Check sheet for the modelled part. Datum: model origin and axes. Units: mm. A direction names the side the tool comes from. Give positions to 0.01 mm unless a question says otherwise; leave off trailing zeros. Loops run counter-clockwise (first coordinate to the right, second up) from the corner with the lowest first, then second, coordinate; pieces in that order, holes last. Notation, with made-up numbers: M 64.5,49.5 L 90.5,49.5 A22 cw 90.5,66.5 Z; hole C -24.5,-6.75 d7. An arc over 180 degrees is marked long. Put each result on its own line as item: value. Start each with the question number.
```python
from build123d import *

# Parameters (mm, degrees)
SKETCH3_R           = 0.9
SKETCH3_W           = 4.2
SKETCH3_H           = 8
SKETCH3_H_2         = 6
BOSS_EXTRUDE3_DEPTH = 2


with BuildPart() as part:
    # Sketch3 → Boss-Extrude3 (new body)
    with BuildSketch(Plane.XY):
        with BuildLine():
            Line((0, 94.006448831), (0, 86.061448831))
            ThreePointArc((0, 86.061448831), (0.585786438, 84.647235269), (2, 84.061448831))
            Line((2, 84.061448831), (4, 84.061448831))
            Line((4, 84.061448831), (4, 78.061448831))
            Line((4, 78.061448831), (2, 78.061448831))
            ThreePointArc((2, 78.061448831), (0.585786438, 77.475662393), (0, 76.061448831))
            Line((0, 76.061448831), (0, 60.606448831))
            ThreePointArc((0, 60.606448831), (0.585786438, 59.192235269), (2, 58.606448831))
            Line((2, 58.606448831), (4, 58.606448831))
            Line((4, 58.606448831), (4, 50.606448831))
            Line((4, 50.606448831), (2, 50.606448831))
            ThreePointArc((2, 50.606448831), (0.585786438, 50.020662393), (0, 48.606448831))
            Line((0, 48.606448831), (0, 26.346448831))
            ThreePointArc((0, 26.346448831), (0.585786438, 24.932235269), (2, 24.346448831))
            Line((2, 24.346448831), (4, 24.346448831))
            Line((4, 24.346448831), (4, 12.346448831))
            Line((4, 12.346448831), (6, 12.346448831))
            Line((6, 12.346448831), (6, 24.346448831))
            Line((6, 24.346448831), (10.2, 24.346448831))
            Line((10.2, 24.346448831), (10.2, 12.346448831))
            Line((10.2, 12.346448831), (12.2, 12.346448831))
            Line((12.2, 12.346448831), (12.2, 24.346448831))
            Line((12.2, 24.346448831), (14.2, 24.346448831))
            ThreePointArc((14.2, 24.346448831), (15.614213562, 24.932235269), (16.2, 26.346448831))
            Line((16.2, 26.346448831), (16.2, 48.606448831))
            ThreePointArc((16.2, 48.606448831), (15.614213562, 50.020662393), (14.2, 50.606448831))
            Line((14.2, 50.606448831), (12.2, 50.606448831))
            Line((12.2, 50.606448831), (12.2, 58.606448831))
            Line((12.2, 58.606448831), (14.2, 58.606448831))
            ThreePointArc((14.2, 58.606448831), (15.614213562, 59.192235269), (16.2, 60.606448831))
            Line((16.2, 60.606448831), (16.2, 76.061448831))
            ThreePointArc((16.2, 76.061448831), (15.614213562, 77.475662393), (14.2, 78.061448831))
            Line((14.2, 78.061448831), (12.2, 78.061448831))
            Line((12.2, 78.061448831), (12.2, 84.061448831))
            Line((12.2, 84.061448831), (14.2, 84.061448831))
            ThreePointArc((14.2, 84.061448831), (15.614213562, 84.647235269), (16.2, 86.061448831))
            Line((16.2, 86.061448831), (16.2, 94.006448831))
            Line((16.2, 94.006448831), (0, 94.006448831))
        make_face()
        with Locations((6, 33.846448831)):
            Circle(SKETCH3_R, mode=Mode.SUBTRACT)
        with Locations((10.2, 33.846448831)):
            Circle(SKETCH3_R, mode=Mode.SUBTRACT)
        with Locations((2.75, 86.061448831)):
            Circle(SKETCH3_R, mode=Mode.SUBTRACT)
        with Locations((10.2, 41.166448831)):
            Circle(SKETCH3_R, mode=Mode.SUBTRACT)
        with Locations((13.45, 48.106448831)):
            Circle(SKETCH3_R, mode=Mode.SUBTRACT)
        with Locations((2.75, 92.061448831)):
            Circle(SKETCH3_R, mode=Mode.SUBTRACT)
        with Locations((13.45, 86.061448831)):
            Circle(SKETCH3_R, mode=Mode.SUBTRACT)
        with Locations((2.75, 61.106448831)):
            Circle(SKETCH3_R, mode=Mode.SUBTRACT)
        with Locations((13.45, 61.106448831)):
            Circle(SKETCH3_R, mode=Mode.SUBTRACT)
        with Locations((2.75, 75.561448831)):
            Circle(SKETCH3_R, mode=Mode.SUBTRACT)
        with Locations((13.45, 26.846448831)):
            Circle(SKETCH3_R, mode=Mode.SUBTRACT)
        with Locations((13.45, 75.561448831)):
            Circle(SKETCH3_R, mode=Mode.SUBTRACT)
        with Locations((13.45, 92.061448831)):
            Circle(SKETCH3_R, mode=Mode.SUBTRACT)
        with Locations((2.75, 26.846448831)):
            Circle(SKETCH3_R, mode=Mode.SUBTRACT)
        with Locations((6, 41.106448831)):
            Circle(SKETCH3_R, mode=Mode.SUBTRACT)
        with Locations((2.75, 48.106448831)):
            Circle(SKETCH3_R, mode=Mode.SUBTRACT)
        with Locations((8.1, 54.606448831)):
            Rectangle(SKETCH3_W, SKETCH3_H, mode=Mode.SUBTRACT)
        with Locations((8.1, 81.061448831)):
            Rectangle(SKETCH3_W, SKETCH3_H_2, mode=Mode.SUBTRACT)
    extrude(amount=BOSS_EXTRUDE3_DEPTH)


solid = part.part
```
Q1. Mould release check, pull along X, two halves, no side actions. Record for faces 1 (the face through (12.2, 55, 1)), 2 (the face through (10.2, 18, 1)), 3 (the face through (3.23, 48.87, 0.99)), 4 (the face through (4.4, 53.7, 2)): pulls with the +X half, pulls with the -X half, needs draft (parallel to the pull), parting line crosses it, or undercut.
Q2. Access from +Z, -Z, +X, -X, +Y, -Y to the whole of each face (thin tool, end or side, straight path). Record for faces 5 (the face through (4, 81, 1)), 6 (the face through (15.63, 50.005, 0.986)), 7 (the face through (10.2, 55, 1)), 8 (the face through (16.2, 90, 1)), 9 (the face through (4, 18, 1)).
Q3. Section check A-A, the plane y = 22. Record the cut outline in (x, z).
Q4. Section check B-B, the plane x = 2.75. Give the number of separate pieces and of enclosed holes in the cut face, then the cut area to 3 significant figures.
Q5. Thickness scan on line 1 along Y through (x, z) = (8, 1.75); line 2 along X through (y, z) = (16.5, 1); line 3 along Y through (x, z) = (10, 1.4). Record the ranges inside material, lowest first. Write a range as [from, to].
Q6. Depth check by flat-ended pin: P1, Ø1, axis at x = 3, z = 1, coming from the -Y side; P2, Ø0.6, axis at y = 55, z = 1, coming from the -X side; P3, Ø1.4, axis at x = 2.75, y = 48.11, coming from the +Z side; P4, Ø3, axis at x = 13.45, y = 86.06, coming from the -Z side. Enter the tip coordinate at first touch or a pass-through.
Found:
1. face 1: pulls with the +X half
1. face 2: undercut
1. face 3: undercut
1. face 4: needs draft
2. face 5: +Z, -Z, -X
2. face 6: +Z, -Z, +X
2. face 7: +Z, -Z
2. face 8: +Z, -Z, +X, +Y, -Y
2. face 9: +Z, -Z, -X, -Y
3. outline: M 4,0 L 6,0 L 6,2 L 4,2 Z; M 10.2,0 L 12.2,0 L 12.2,2 L 10.2,2 Z
4. separate pieces: 9
4. enclosed holes: 0
4. area: 89.7 mm^2
5. line 1: y = [24.35, 50.61], [58.61, 78.06], [84.06, 94.01]
5. line 2: x = [4, 6], [10.2, 12.2]
5. line 3: y = [24.35, 32.97], [34.72, 40.29], [42.04, 50.61], [58.61, 78.06], [84.06, 94.01]
6. P1: stops at y = 24.35
6. P2: stops at x = 4
6. P3: passes through
6. P4: stops at z = 0
